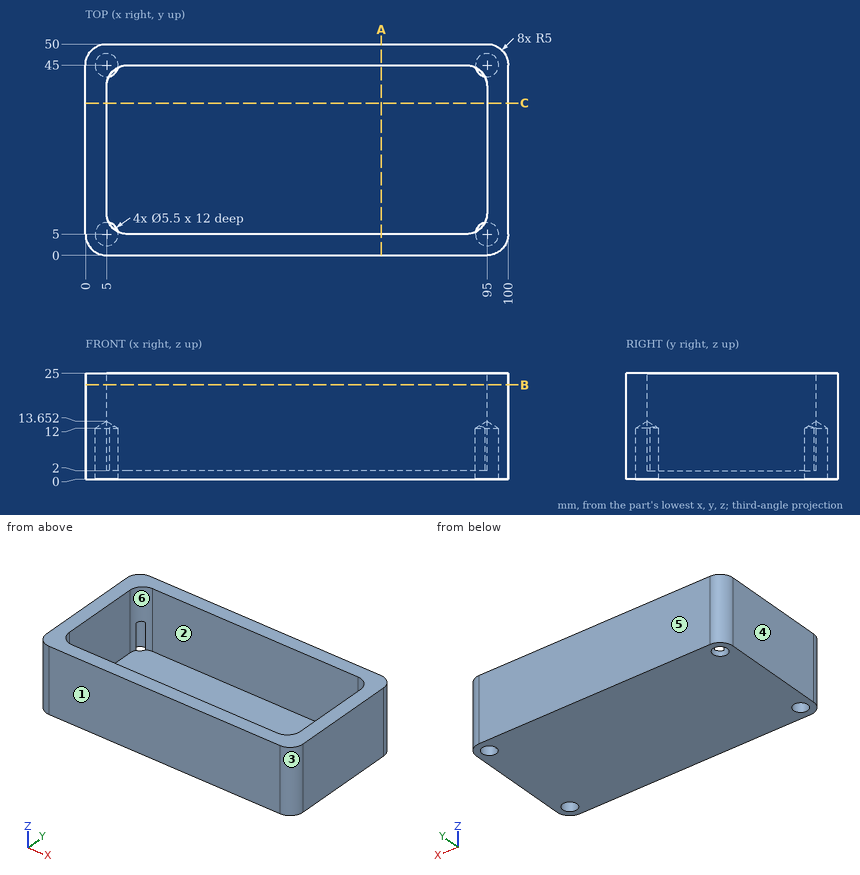
For this review, use the dimensioned drawing (mm, ordinates from the lowest corner) and the shaded views. A direction names the side the tool comes from. Give positions to 0.01 mm unless a question says otherwise; leave off trailing zeros. Order: outer loops, then holes, each group sorted by start corner. A loop starts at its lowest first (then second) coordinate and runs counter-clockwise, first axis right, second up.
1. Add section B-B, the plane z = 22.25. State the section outline as (x, y) points, then the cut area to 3 significant figures.
Solution:
outline: (0, 5) arc R5 ccw to (5, 0) - (95, 0) arc R5 ccw to (100, 5) - (100, 45) arc R5 ccw to (95, 50) - (5, 50) arc R5 ccw to (0, 45) - close; hole (5, 10) arc R5 ccw to (10, 5) - (90, 5) arc R5 ccw to (95, 10) - (95, 40) arc R5 ccw to (90, 45) - (10, 45) arc R5 ccw to (5, 40) - close
area: 1,400 mm2
2. Add section A-A, the plane x = 70. State the section outline as (y, z) points, then the cut area to 3 significant figures.
Solution:
outline: (0, 0) - (50, 0) - (50, 25) - (45, 25) - (45, 2) - (5, 2) - (5, 25) - (0, 25) - close
area: 330 mm2
3. For pin 1 Ø11.5 at (y, z) = (21, 19) entering from -X; pin 2 Ø8 at (x, y) = (27, 38.5) entering from +Z; pin 3 Ø3.5 at (x, y) = (5, 5) entering from -Z, all flat-tipped, find the tip position at first contact; note any pin that passes through.
Solution:
pin 1: stops at x = 0
pin 2: stops at z = 2
pin 3: stops at z = 12.6
4. Tool access review of the marked faces 1 and 2: name each direction out of +Z, -Z, +X, -X, +Y, -Y from which nothing blocks a thin tool from reaching the whole face with its end or side.
Solution:
face 1: +Z, -Z, +X, -X, -Y
face 2: +Z
5. To check wall thickness, follow L1, parallel to X at y = 15.5, z = 18.75; L2, parallel to Y at x = 48, z = 18.5; L3, parallel to X at y = 44, z = 12.5 (1 decimal). State the ranges of each line that lie inside material, in increasing order.
Solution:
L1: x = 0 to 5, 95 to 100
L2: y = 0 to 5, 45 to 50
L3: x = 0 to 3.4, 6.6 to 7, 93 to 93.4, 96.6 to 100
6. Add section C-C, the plane y = 36. State the section outline as (x, z) points.
Solution:
outline: (0, 0) - (100, 0) - (100, 25) - (95, 25) - (95, 2) - (5, 2) - (5, 25) - (0, 25) - close
7. Mouldability with a two-part tool opening along Y and no side actions: class the marked faces 3, 4, 5 and 6 as +Y half, -Y half, draft (parallel to the pull), parting line (faces both ways), or undercut.
Solution:
face 3: -Y half
face 4: draft
face 5: +Y half
face 6: undercut
